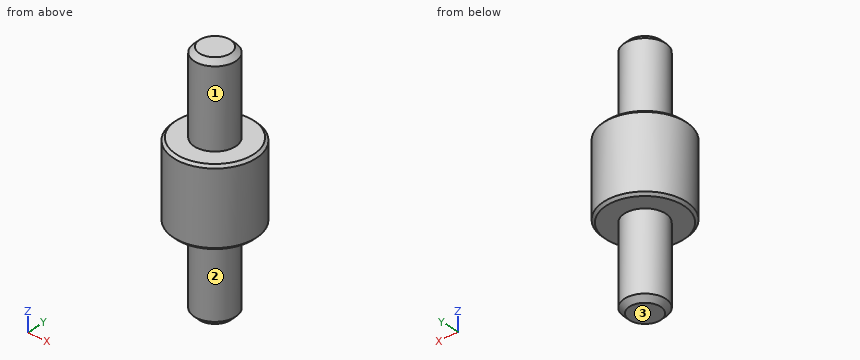
```python
from build123d import *

# Parameters (mm, degrees)
F2_SIZE = 0.5
F3_SIZE = 1


with BuildPart() as f1:
    # F0 (on Front) → F1 (revolve)
    with BuildSketch(Plane.XZ):
        Polygon((0, 47), (0, 0), (4, 0), (4, 16), (8, 16), (8, 31), (4, 31), (4, 47), align=None)
    revolve(axis=Axis((0, 0, 23.5), (0, 0, 1)))

    # F2
    f2_edges = [f1.edges().sort_by_distance(p)[0] for p in [
        (-8, 0, 31),
        (-8, 0, 16),
    ]]
    chamfer(f2_edges, length=F2_SIZE)

    # F3
    f3_edges = [f1.edges().sort_by_distance(p)[0] for p in [
        (-4, 0, 47),
        (-4, 0, 0),
    ]]
    chamfer(f3_edges, length=F3_SIZE)


solid = f1.part
```
The model under review builds one solid part; all positions refer to its coordinate system, in mm. Face numbers are marked on the shaded views. A direction names the side the tool comes from. Round coordinates to 2 decimals unless told otherwise and drop trailing zeros. Order: outer loops, then holes, each group sorted by start corner. A loop starts at its lowest first (then second) coordinate and runs counter-clockwise, first axis right, second up. Notation, with made-up numbers: (-4, 24) - (18, 24) arc R9 cw to (18, 30) - close; hole circle Ø10 at (-38.5, 31.25). An arc over 180 degrees is marked (long way). Answer in a Markdown table with one row per item.
(1) Machinability: for the marked faces 1, 2 and 3, which of the approach directions +Z, -Z, +X, -X, +Y, -Y give a long, thin tool a straight path to every point of the face, cutting with its end or side? Answer none if there is none.
Result set:
| item | result |
|---|---|
| face 1 | +Z |
| face 2 | -Z |
| face 3 | -Z, +X, -X, +Y, -Y |
(2) Clearance check with flat-ended pins moving along their axes: P1, Ø3, axis at x = 1.5, z = 7.5, coming from the +Y side; P2, Ø6, axis at x = 1, z = 11.5, coming from the -Y side; P3, Ø7.5, axis at x = -1, y = -2.5, coming from the -Z side; P4, Ø2, axis at x = -1, y = 4.5, coming from the -Z side. State where each tip first meets the part, or that it passes through.
Result set:
| item | result |
|---|---|
| P1 | stops at y = 4 |
| P2 | stops at y = -4 |
| P3 | stops at z = 0 |
| P4 | stops at z = 0.61 |
(3) Take a section at C-C on z = 39. Write out the cut boundary in (x, y), plus the area to 3 significant figures.
Result set:
| item | result |
|---|---|
| outline | circle Ø8 at (0, 0) |
| area | 50.3 mm2 |
(4) Take a section at A-A on x = 0. Write out the cut boundary in (y, z).
Result set:
| item | result |
|---|---|
| outline | (-8, 16.5) - (-7.5, 16) - (-4, 16) - (-4, 1) - (-3, 0) - (3, 0) - (4, 1) - (4, 16) - (7.5, 16) - (8, 16.5) - (8, 30.5) - (7.5, 31) - (4, 31) - (4, 46) - (3, 47) - (-3, 47) - (-4, 46) - (-4, 31) - (-7.5, 31) - (-8, 30.5) - close |
(5) Take a section at D-D on z = 26. Write out the cut boundary in (x, y).
Result set:
| item | result |
|---|---|
| outline | circle Ø16 at (0, 0) |
(6) For line 1 (Z direction, x = -3.75, y = 6.5); line 2 (X direction, y = 0.75, z = 41), list the stretches that pass through material, from the lowest coordinate up. Write a range as from..to.
Result set:
| item | result |
|---|---|
| line 1 | z = 16..31 |
| line 2 | x = -3.93..3.93 |
